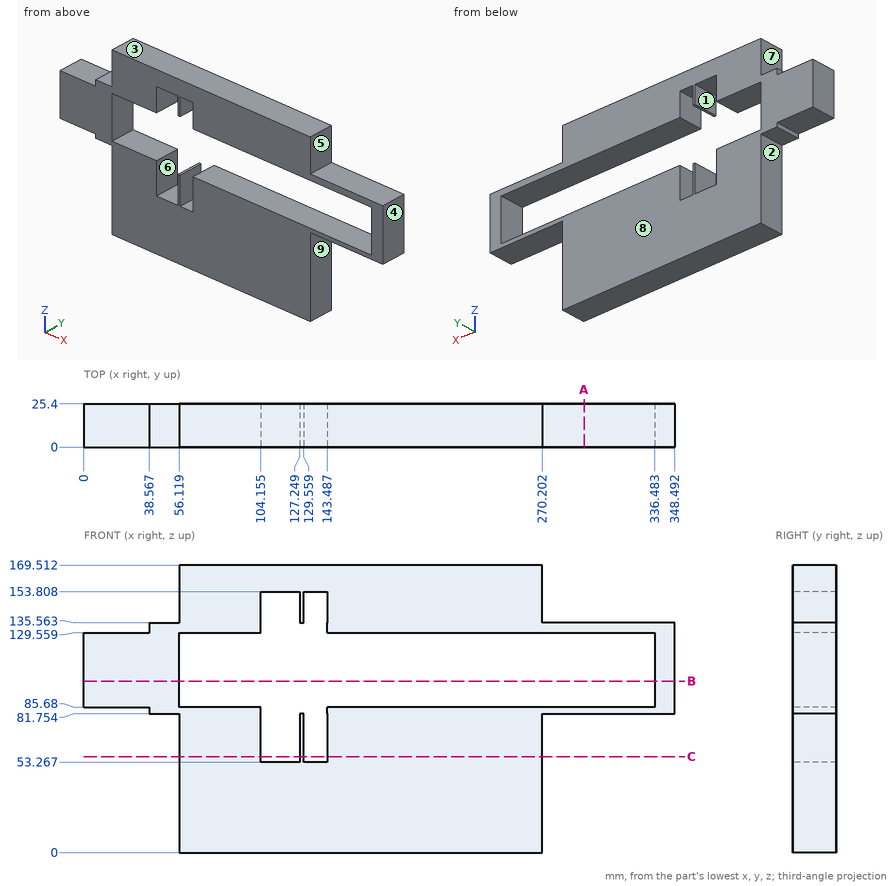
Could you check a few things on this drawing? It's one solid part, dimensions in mm from its lowest x, y, z. A direction names the side the tool comes from. Give positions to 0.01 mm unless a question says otherwise; leave off trailing zeros. Write each loop counter-clockwise with the first axis right and the second up, starting at its lowest first coordinate (ties: lowest second). Pieces come first, ordered by that corner, then holes. Notation, with made-up numbers: (15, 75.25) -> (61, 75.25) arc R33 ccw to (61, 112.25) -> close; hole circle Ø3 at (84.25, -2). An arc over 180 degrees is marked (long way). Write each question's results on one line, items separated by ' | '.
1. Will these pins go through, and if not, where does the flat tip stop? pin 1 Ø7.5 at (y, z) = (16.5, 38) entering from -X; pin 2 Ø5 at (y, z) = (4, 23) entering from +X; pin 3 Ø12.5 at (x, y) = (314.5, 12.5) entering from +Z.
Check sheet entries:
pin 1: stops at x = 56.12 | pin 2: stops at x = 270.2 | pin 3: stops at z = 135.56
2. I want a section at B-B, the plane z = 101. Write out the boundary of the cut face in (x, y), then the cut area to 3 significant figures.
Check sheet entries:
outline: (0, 0) -> (56.12, 0) -> (56.12, 25.4) -> (0, 25.4) -> close; (336.48, 0) -> (348.49, 0) -> (348.49, 25.4) -> (336.48, 25.4) -> close | area: 1,730 mm²
3. I need wall thicknesses on L1, parallel to Z at x = 231.5, y = 6; L2, parallel to X at y = 5, z = 121; L3, parallel to X at y = 16, z = 84 (1 decimal). Which ranges of each line are inside material? Lowest first, please.
Check sheet entries:
L1: z = 0 to 85.68, 129.56 to 169.51 | L2: x = 0 to 56.12, 336.48 to 348.49 | L3: x = 38.6 to 104.2, 143.5 to 348.5
4. On a 3-axis mill with a long thin cutter (end or side, diameter ignored), from which of +Z, -Z, +X, -X, +Y, -Y can I reach the whole of each face in a straight line? I mean the marked faces 5, 6, 7, 8 and 9. Say none if no direction works.
Check sheet entries:
face 5: +Z, +X, +Y, -Y | face 6: +Y, -Y | face 7: +Z, -X, +Y, -Y | face 8: +Z, -Z, +X, -X, +Y | face 9: -Z, +X, +Y, -Y
5. I want a section at C-C, the plane z = 56.5. Count the separate pieces of the cut face and the enclosed holes in it, then the cut area to 3 significant figures.
Check sheet entries:
separate pieces: 3 | enclosed holes: 0 | area: 4,500 mm²
6. If we mould it in two halves opening along X, with no side actions, what happens to the marked faces 1, 2, 3 and 4? For each: released by +X, released by -X, zero draft, split by the parting line, or undercut.
Check sheet entries:
face 1: undercut | face 2: released by -X | face 3: zero draft | face 4: released by +X
7. I want a section at A-A, the plane x = 295. Write out the boundary of the cut face in (y, z).
Check sheet entries:
outline: (0, 81.75) -> (25.4, 81.75) -> (25.4, 85.68) -> (0, 85.68) -> close; (0, 129.56) -> (25.4, 129.56) -> (25.4, 135.56) -> (0, 135.56) -> close
